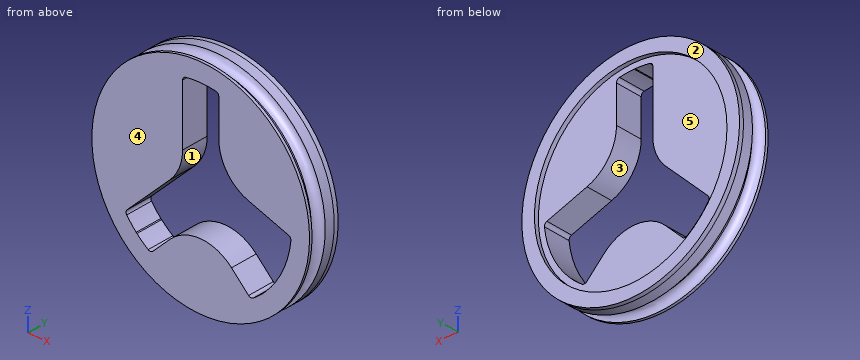
from build123d import *

# Parameters (mm, degrees)
F0_R     = 19.05
F1_DEPTH = 4.7625
F3_DEPTH = 25.4
F4_R     = 0.635
F5_R     = 7.62
F6_R     = 19.05
F6_R_2   = 16.8477682608
F7_DEPTH = 0.762
F8_R     = 1.27


with BuildPart() as f1:
    # F0 (on Front) → F1 (new body)
    with BuildSketch(Plane.XZ):
        Circle(F0_R)
    extrude(amount=F1_DEPTH)

    # F2 (on face) → F3 (cut)
    with BuildSketch(Plane.XZ.offset(4.7625)):
        with BuildLine():
            ThreePointArc((-13.2419744131, -8.7555045953), (-12.3238425839, -10.0067993588), (-11.2879133137, -11.1624615879))
            ThreePointArc((-11.2879133137, -11.1624615879), (-11.2235221627, -11.2272144784), (-11.1587595957, -11.2915958968))
            ThreePointArc((-11.1587595957, -11.2915958968), (-10.0029416889, -12.32735147), (-8.7515089527, -13.2452952306))
            Line((-8.7515089527, -13.2452952306), (0.0012918382, -4.4911788753))
            Line((0.0012918382, -4.4911788753), (8.7554081934, -13.2439796662))
            ThreePointArc((8.7554081934, -13.2439796662), (10.006702957, -12.325847837), (11.1623651861, -11.2899185668))
            ThreePointArc((11.1623651861, -11.2899185668), (11.2271180766, -11.2255274158), (11.291499495, -11.1607648488))
            ThreePointArc((11.291499495, -11.1607648488), (14.4575372164, -6.5602305791), (15.8344708919, -1.1479515698))
            Line((15.8344708919, -1.1479515698), (3.1757157521, 3.1741877502))
            Line((3.1757157521, 3.1741877502), (3.1747959638, 15.4156336391))
            Line((3.1747959638, 15.4156336391), (3.1747856088, 15.5534475772))
            ThreePointArc((3.1747856088, 15.5534475772), (1.6407693424, 15.7890293509), (0.0910801197, 15.8736933393))
            ThreePointArc((0.0910801197, 15.8736933393), (-0.0002385077, 15.8739491277), (-0.0915570956, 15.8736796149))
            ThreePointArc((-0.0915570956, 15.8736796149), (-1.6412335946, 15.7887827216), (-3.1752144554, 15.5529703966))
            Line((-3.1752144554, 15.5529703966), (-3.1741441565, 1.3138388775))
            Line((-3.1741441565, 1.3138388775), (-13.2419744131, -8.7555045953))
        make_face()
        with BuildLine():
            Line((-3.1740454005, 0), (-3.1741441565, 1.3138388775))
            Line((-3.1741441565, 1.3138388775), (-2.2442783045, 2.2438444902))
            ThreePointArc((-2.2442783045, 2.2438444902), (-2.9322076505, 1.2143442667), (-3.1740454005, 0))
        make_face(mode=Mode.SUBTRACT)
        with BuildLine():
            Line((-2.2442783045, 2.2438444902), (-3.1741441565, 1.3138388775))
            Line((-3.1741441565, 1.3138388775), (-3.1740454005, 0))
            ThreePointArc((-3.1740454005, 0), (-2.9322076505, 1.2143442667), (-2.2442783045, 2.2438444902))
        make_face()
        with BuildLine():
            ThreePointArc((-11.1587595957, -11.2915958968), (-11.2235221627, -11.2272144784), (-11.2879133137, -11.1624615879))
            ThreePointArc((-11.2879133137, -11.1624615879), (-11.2242651795, -11.2279576068), (-11.1587595957, -11.2915958968))
        make_face()
        with BuildLine():
            ThreePointArc((0.0910801197, 15.8736933393), (-0.0002385867, 15.874999991), (-0.0915570956, 15.8736796149))
            ThreePointArc((-0.0915570956, 15.8736796149), (-0.0002385077, 15.8739491277), (0.0910801197, 15.8736933393))
        make_face()
        with BuildLine():
            ThreePointArc((11.291499495, -11.1607648488), (11.2271180766, -11.2255274158), (11.1623651861, -11.2899185668))
            ThreePointArc((11.1623651861, -11.2899185668), (11.227861205, -11.2262704326), (11.291499495, -11.1607648488))
        make_face()
    extrude(amount=-F3_DEPTH, mode=Mode.SUBTRACT)

    # F4
    f4_edges = [f1.edges().sort_by_distance(p)[0] for p in [
        (-13.241974, -2.38125, -8.755505),
        (-8.751509, -2.38125, -13.245295),
        (8.755408, -2.38125, -13.24398),
        (15.834471, -2.38125, -1.147952),
        (3.174786, -2.38125, 15.553448),
        (-3.175214, -2.38125, 15.55297),
    ]]
    fillet(f4_edges, radius=F4_R)

    # F5
    f5_edges = [f1.edges().sort_by_distance(p)[0] for p in [
        (-3.174144, -2.38125, 1.313839),
        (0.001292, -2.38125, -4.491179),
        (3.175716, -2.38125, 3.174188),
    ]]
    fillet(f5_edges, radius=F5_R)

    # F6 (on face) → F7 (join)
    with BuildSketch(Plane(origin=(0, 0, 0), x_dir=(-1, 0, 0), z_dir=(0, 1, 0))):
        Circle(F6_R)
        Circle(F6_R_2, mode=Mode.SUBTRACT)
    extrude(amount=F7_DEPTH)

    # F8 (on Top) → F9 (revolve, cut)
    with BuildSketch(Plane.XY):
        with Locations((-19.0806053579, -3.0079341959)):
            Circle(F8_R)
    revolve(axis=Axis((0, 0.762, 0), (0, 1, 0)), mode=Mode.SUBTRACT)


solid = f1.part
Read the model definition and answer for the solid it produces. Units are mm, in the model's axes. Face numbers are marked on the shaded views. A direction names the side the tool comes from. Give positions to 0.01 mm unless a question says otherwise; leave off trailing zeros. Write each loop counter-clockwise with the first axis right and the second up, starting at its lowest first coordinate (ties: lowest second). Pieces come first, ordered by that corner, then holes. Notation, with made-up numbers: (-32.75, 53) - (-14.75, 53) arc R25 cw to (-14.75, 92) - close; hole circle Ø10 at (27, -30.75). An arc over 180 degrees is marked (long way). Return JSON: item names as keys, results as strings.
Q1. For the marked faces 3, 4 and 5, determine the directions among +Z, -Z, +X, -X, +Y, -Y from which every point of the face is accessible in a straight line to the end or side of a thin tool.
Reply:
{"face 3": "+Y, -Y", "face 4": "+Z, -Z, +X, -X, -Y", "face 5": "+Y"}
Q2. A cutting plane is placed at A-A, the plane z = 0. Determine the outline of the cut face in (x, y).
Reply:
{"outline": "(-19.05, -4.76) - (-4.62, -4.76) - (-4.62, 0) - (-16.85, 0) - (-16.85, 0.76) - (-19.05, 0.76) - (-19.05, -1.74) arc R1.27 cw to (-19.05, -4.28) - close; (12.47, -4.76) - (19.05, -4.76) - (19.05, -4.28) arc R1.27 cw to (19.05, -1.74) - (19.05, 0.76) - (16.85, 0.76) - (16.85, 0) - (12.47, 0) - close"}
Q3. For a pull along X with two mould halves and no side action, classify the marked faces 1 and 2 as released by +X, released by -X, zero draft, split by the parting line, or undercut.
Reply:
{"face 1": "undercut", "face 2": "zero draft"}
Q4. Given P1, Ø1.4, axis at y = -1.5, z = 13.5, coming from the -X side; P2, Ø10, axis at x = 2.5, z = 1.5, coming from the +Y side; P3, Ø2.5, axis at y = -3.5, z = 11, coming from the +X side, each flat-ended and moving along its own axis, determine where each tip first touches the part or whether it passes through.
Reply:
{"P1": "x = -14.11", "P2": "y = 0", "P3": "x = 16.2"}
Q5. Consider line 1 along Z through (x, y) = (0, 0.6); line 2 along Y through (x, z) = (7, -13); line 3 along Z through (x, y) = (4, -3.7). Determine where each line is inside the solid, lowest interval first. Write a range as [from, to].
Reply:
{"line 1": "[-19.05, -16.85], [16.85, 19.05]", "line 2": "[-4.76, 0]", "line 3": "[-17.57, -8.78], [5.18, 17.57]"}
